```python
from build123d import *

# Parameters (mm, degrees)
SKETCH1_R           = 21.5
SKETCH1_R_2         = 15.5
BOSS_EXTRUDE1_DEPTH = 4
BOSS_EXTRUDE2_START = 4
SKETCH2_R           = 21.5
SKETCH2_R_2         = 18.5
BOSS_EXTRUDE2_DEPTH = 4
SKETCH3_R           = 18.5
SKETCH3_R_2         = 15
CUT_EXTRUDE1_DEPTH  = 2
SKETCH4_R           = 2
BOSS_EXTRUDE3_DEPTH = 4
FILLET1_R           = 10
CUT_EXTRUDE3_DEPTH  = 1


with BuildPart() as part:
    # Sketch1 → Boss-Extrude1 (new body)
    with BuildSketch(Plane(origin=(0, 0, 0), x_dir=(1, 0, 0), z_dir=(0, 1, 0))):
        with Locations(Location((0, 0, 0), (0, 0, 270))):
            Circle(SKETCH1_R)
        with Locations(Location((0, 0, 0), (0, 0, 270))):
            Circle(SKETCH1_R_2, mode=Mode.SUBTRACT)
    extrude(amount=BOSS_EXTRUDE1_DEPTH)

    # Sketch2 → Boss-Extrude2 (add)
    with BuildSketch(Plane.XZ.offset(BOSS_EXTRUDE2_START)):
        with Locations(Location((0, 0, 0), (0, 0, 270))):
            Circle(SKETCH2_R)
        with Locations(Location((0, 0, 0), (0, 0, 270))):
            Circle(SKETCH2_R_2, mode=Mode.SUBTRACT)
    extrude(amount=-BOSS_EXTRUDE2_DEPTH)

    # Sketch3 → Cut-Extrude1 (cut)
    with BuildSketch(Plane.XZ):
        with Locations(Location((0, 0, 0), (0, 0, 270))):
            Circle(SKETCH3_R)
        Circle(SKETCH3_R_2, mode=Mode.SUBTRACT)
    extrude(amount=-CUT_EXTRUDE1_DEPTH, mode=Mode.SUBTRACT)

    # Sketch4 → Boss-Extrude3 (add)
    # profile 1 of 4: a face of its own
    with BuildSketch(Plane.XZ.offset(4)):
        with BuildLine():
            Line((-25.5, 4), (-20.187008248, 4))
            Line((-20.187008248, 4), (-20.187008248, -4))
            Line((-20.187008248, -4), (-25.5, -4))
            ThreePointArc((-25.5, -4), (-29.5, 0), (-25.5, 4))
        make_face()
        with Locations(Location((-25.5, 0, 0), (0, 0, 270))):
            Circle(SKETCH4_R, mode=Mode.SUBTRACT)
    # profile 2 of 4: a face of its own
    with BuildSketch(Plane.XZ.offset(4)):
        with BuildLine():
            Line((4, 20.187008248), (-4, 20.187008248))
            Line((-4, 20.187008248), (-4, 25.5))
            ThreePointArc((-4, 25.5), (0, 29.5), (4, 25.5))
            Line((4, 25.5), (4, 20.187008248))
        make_face()
        with Locations(Location((0, 25.5, 0), (0, 0, 270))):
            Circle(SKETCH4_R, mode=Mode.SUBTRACT)
    # profile 3 of 4: a face of its own
    with BuildSketch(Plane.XZ.offset(4)):
        with BuildLine():
            Line((20.187008248, -4), (20.187008248, 4))
            Line((20.187008248, 4), (25.5, 4))
            ThreePointArc((25.5, 4), (29.5, 0), (25.5, -4))
            Line((25.5, -4), (20.187008248, -4))
        make_face()
        with Locations(Location((25.5, 0, 0), (0, 0, 270))):
            Circle(SKETCH4_R, mode=Mode.SUBTRACT)
    # profile 4 of 4: a face of its own
    with BuildSketch(Plane.XZ.offset(4)):
        with BuildLine():
            Line((-4, -20.187008248), (4, -20.187008248))
            Line((4, -20.187008248), (4, -25.5))
            ThreePointArc((4, -25.5), (0, -29.5), (-4, -25.5))
            Line((-4, -25.5), (-4, -20.187008248))
        make_face()
        with Locations(Location((0, -25.5, 0), (0, 0, 270))):
            Circle(SKETCH4_R, mode=Mode.SUBTRACT)
    extrude(amount=-BOSS_EXTRUDE3_DEPTH)

    # Fillet1
    # the kernel refuses this fillet: 10 mm, written as the material it adds along each edge
    with BuildSketch(Plane(origin=(-4, 0, 21.124630174), x_dir=(0.016272387136782942, 0, 0.9998675959430181), z_dir=(0, -1, 0)), Plane(origin=(4, 0, -21.124630174), x_dir=(-0.01627238713686073, 0, -0.9998675959430169), z_dir=(0, -1, 0)), Plane(origin=(-21.124630174, 0, -4), x_dir=(-0.9998675959430171, 0, 0.01627238713684981), z_dir=(0, -1, 0)), Plane(origin=(21.124630174, 0, 4), x_dir=(0.9998675959430179, 0, -0.01627238713679413), z_dir=(0, -1, 0))) as fillet1_piece_1:
        with BuildLine():
            CenterArc((7.07924631, 9.82068168), FILLET1_R, 206.72107826, 52.41213662)
            Line((-1.852813991, 5.324205419), (-2.746020021, 4.874557792))
            ThreePointArc((-2.746020021, 4.874557792), (-1.695593605, 2.394427141), (-0.979383425, -0.202010165))
            Line((-0.979383425, -0.202010165), (0.016272387, -0.999867596))
            ThreePointArc((0.016272387, -0.999867596), (4.391062896, -0.928669884), (5.00545854, -0.982068168))
            Line((5.00545854, -0.982068168), (5.193984701, 0))
        make_face()
    extrude(amount=4)
    with BuildSketch(Plane(origin=(-21.124630174, 0, 4), x_dir=(-0.9998675959430171, 0, -0.016272387136849455), z_dir=(0, -1, 0)), Plane(origin=(-4, 0, -21.124630174), x_dir=(0.0162723871369052, 0, -0.9998675959430161), z_dir=(0, -1, 0)), Plane(origin=(21.124630174, 0, -4), x_dir=(0.9998675959430168, 0, 0.016272387136866445), z_dir=(0, -1, 0)), Plane(origin=(4, 0, 21.124630174), x_dir=(-0.0162723871368113, 0, 0.9998675959430178), z_dir=(0, -1, 0))) as fillet1_piece_2:
        with BuildLine():
            CenterArc((7.07924631, -9.82068168), FILLET1_R, 100.86678512, 52.41213662)
            Line((-1.852813991, -5.324205419), (-2.746020021, -4.874557792))
            ThreePointArc((-2.746020021, -4.874557792), (-1.695593605, -2.394427141), (-0.979383425, 0.202010165))
            Line((-0.979383425, 0.202010165), (0.016272387, 0.999867596))
            ThreePointArc((0.016272387, 0.999867596), (4.391062896, 0.928669884), (5.00545854, 0.982068168))
            Line((5.00545854, 0.982068168), (5.193984701, 0))
        make_face()
    extrude(amount=4)

    # Sketch6 → Cut-Extrude3 (cut)
    with BuildSketch(Plane(origin=(0, 4, 0), x_dir=(1, 0, 0), z_dir=(0, 1, 0))):
        Polygon((-8.667268163, 11.849248678), (-15.190647858, 18.372628373), (-18.372628373, 15.190647858), (-11.849248678, 8.667268163), align=None)
    extrude(amount=-CUT_EXTRUDE3_DEPTH, mode=Mode.SUBTRACT)


solid = part.part
```
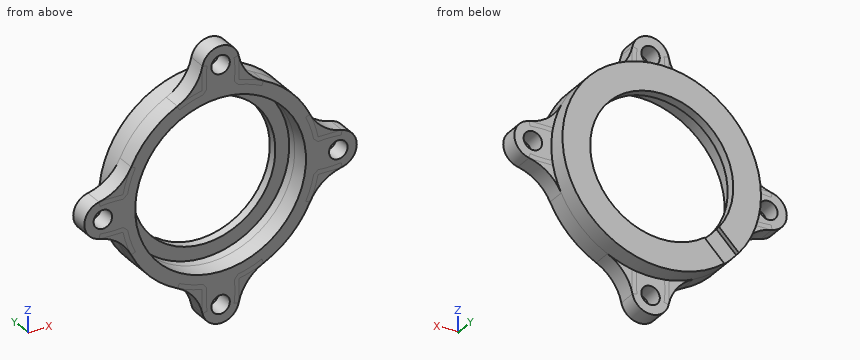
Part model, mm, in its own coordinate system. Round coordinates to 2 decimals unless told otherwise and drop trailing zeros. Loops run counter-clockwise (first coordinate to the right, second up) from the corner with the lowest first, then second, coordinate; pieces in that order, holes last. Notation, with made-up numbers: (14.25, 75.25) -> (32.25, 75.25) arc R11 ccw to (32.25, 81.25) -> close; hole circle Ø7 at (33.5, 9). An arc over 180 degrees is marked (long way). Use a Markdown table: item, result.
1) Cut at C-C, the plane z = 0. List the corners of the cut face in (x, y).
The answers:
| item | result |
|---|---|
| outline | (-29.5, -4) -> (-27.5, -4) -> (-27.5, 0) -> (-29.5, 0) -> close; (-23.5, -4) -> (-18.5, -4) -> (-18.5, 2) -> (-15.5, 2) -> (-15.5, 4) -> (-21.5, 4) -> (-21.5, 0) -> (-23.5, 0) -> close; (15.5, 2) -> (18.5, 2) -> (18.5, -4) -> (23.5, -4) -> (23.5, 0) -> (21.5, 0) -> (21.5, 4) -> (15.5, 4) -> close; (27.5, -4) -> (29.5, -4) -> (29.5, 0) -> (27.5, 0) -> close |
2) Cut at A-A, the plane x = 0. List the corners of the cut face in (y, z), and give its area (3 significant figures).
The answers:
| item | result |
|---|---|
| outline | (-4, -29.5) -> (0, -29.5) -> (0, -27.5) -> (-4, -27.5) -> close; (-4, -23.5) -> (0, -23.5) -> (0, -21.5) -> (4, -21.5) -> (4, -15.5) -> (2, -15.5) -> (2, -18.5) -> (-4, -18.5) -> close; (-4, 18.5) -> (2, 18.5) -> (2, 15.5) -> (4, 15.5) -> (4, 21.5) -> (0, 21.5) -> (0, 23.5) -> (-4, 23.5) -> close; (-4, 27.5) -> (0, 27.5) -> (0, 29.5) -> (-4, 29.5) -> close |
| area | 92.0 mm2 |
3) Cut at D-D, the plane z = 7. List the corners of the cut face in (x, y).
The answers:
| item | result |
|---|---|
| outline | (-20.94, -4) -> (-17.12, -4) -> (-17.12, 2) -> (-13.83, 2) -> (-13.83, 4) -> (-20.33, 4) -> (-20.33, 0) -> (-20.94, 0) -> close; (13.83, 2) -> (17.12, 2) -> (17.12, -4) -> (20.94, -4) -> (20.94, 0) -> (20.33, 0) -> (20.33, 4) -> (13.83, 4) -> close |
4) Cut at B-B, the plane y = -1.5. List the corners of the cut face in (x, z).
The answers:
| item | result |
|---|---|
| outline | (-26.32, -3.92) arc R10 cw to (-19.36, -9.35) arc R21.5 ccw to (-9.35, -19.36) arc R10 cw to (-3.92, -26.32) arc R4 ccw to (3.92, -26.32) arc R10 cw to (9.35, -19.36) arc R21.5 ccw to (19.36, -9.35) arc R10 cw to (26.32, -3.92) arc R4 ccw to (26.32, 3.92) arc R10 cw to (19.36, 9.35) arc R21.5 ccw to (9.35, 19.36) arc R10 cw to (3.92, 26.32) arc R4 ccw to (-3.92, 26.32) arc R10 cw to (-9.35, 19.36) arc R21.5 ccw to (-19.36, 9.35) arc R10 cw to (-26.32, 3.92) arc R4 ccw to start; hole circle Ø4 at (-25.5, 0); hole circle Ø37 at (0, 0); hole circle Ø4 at (0, -25.5); hole circle Ø4 at (0, 25.5); hole circle Ø4 at (25.5, 0) |
5) Drop flat-ended pins along their axis: pin 1 Ø0.9 at (x, z) = (-24.5, 3.5) entering from +Y; pin 2 Ø2 at (x, y) = (-17.5, 2.5) entering from -Z; pin 3 Ø3 at (x, y) = (-19.5, -2) entering from +Z; pin 4 Ø1.6 at (x, z) = (8, -23) entering from +Y. Give the stop position or say it passes through.
The answers:
| item | result |
|---|---|
| pin 1 | stops at y = 0 |
| pin 2 | stops at z = -13.78 |
| pin 3 | stops at z = 11.76 |
| pin 4 | passes through |
6) Probe line 1 (X direction, y = -1.8, z = 0); line 2 (X direction, y = 0.55, z = 0); line 3 (Z direction, x = 0, y = 3.65). List the from-to ranges inside material, lowest first. Write a range as [from, to].
The answers:
| item | result |
|---|---|
| line 1 | x = [-29.5, -27.5], [-23.5, -18.5], [18.5, 23.5], [27.5, 29.5] |
| line 2 | x = [-21.5, -18.5], [18.5, 21.5] |
| line 3 | z = [-21.5, -15.5], [15.5, 21.5] |
